Can you work these out from the model? Positions are in its coordinate system, mm. A direction names the side the tool comes from. Give positions to 0.01 mm unless a question says otherwise; leave off trailing zeros. Order: outer loops, then holes, each group sorted by start corner. A loop starts at its lowest first (then second) coordinate and runs counter-clockwise, first axis right, second up. Notation, with made-up numbers: (44.25, -19) -> (96.25, -19) arc R28 cw to (96.25, 8) -> close; hole circle Ø6 at (-40, 35.25). An arc over 180 degrees is marked (long way). Answer as a JSON object with one key per item and string values.
Autodesk Inventor part; units mm, degrees
ref_plane "YZ Plane" through (0, 0, 0) normal (1, 0, 0) x (0, 1, 0)
ref_plane "XZ Plane" through (0, 0, 0) normal (0, 1, 0) x (-1, 0, 0)
ref_plane "XY Plane" through (0, 0, 0) normal (0, 0, 1) x (1, 0, 0)
sketch "스케치1" plane through (0, 0, 0) normal (1, 0, 0) x (0, 1, 0)
  circle A0 centre (0, 0) radius 37
  circle A1 centre (0, 0) radius 4
  dimension "d0" = 74
  dimension "d1" = 8
extrude "돌출1" add sketch "스케치1" along normal blind 24
sketch "스케치2" plane through (24, 0, 0) normal (1, 0, 0) x (0, 0, -1)
  circle A0 centre (0, 0) radius 16
  dimension "d4" = 32
extrude "돌출2" cut sketch "스케치2" against normal blind 19
sketch "스케치4" plane through (5, 0, 0) normal (1, 0, 0) x (0, 0, -1)
  circle A0 centre (0, 10) radius 1.75
  circle A1 centre (10, 0) radius 1.75
  circle A2 centre (0, -10) radius 1.75
  circle A3 centre (-10, 0) radius 1.75
  point P0 (0, 0)
  dimension "d8" = 3.5
  dimension "d9" = 3.5
  dimension "d10" = 3.5
  dimension "d11" = 3.5
extrude "돌출3" cut sketch "스케치4" against normal blind 19
sketch "스케치5" plane through (24, 0, 0) normal (1, 0, 0) x (0, 0, -1)
  circle A0 centre (0, 0) radius 19
  circle A1 centre (0, 0) radius 32
  line L0 (-19.4142, 16.5858) -> (-14.7746, 11.9462)
  line L1 (-23.9974, 21.169) -> (-19.4142, 16.5858)
  line L2 (-16.5858, 19.4142) -> (-11.9462, 14.7746)
  line L3 (-16.5858, 19.4142) -> (-21.169, 23.9974)
  line L4 (16.5858, 19.4142) -> (11.9462, 14.7746)
  line L5 (16.5858, 19.4142) -> (21.169, 23.9974)
  line L6 (19.4142, 16.5858) -> (23.9974, 21.169)
  line L7 (19.4142, 16.5858) -> (14.7746, 11.9462)
  line L8 (16.5858, -19.4142) -> (11.9462, -14.7746)
  line L9 (16.5858, -19.4142) -> (21.169, -23.9974)
  line L10 (19.4142, -16.5858) -> (14.7746, -11.9462)
  line L11 (19.4142, -16.5858) -> (23.9974, -21.169)
  line L12 (-19.4142, -16.5858) -> (-14.7746, -11.9462)
  line L13 (-19.4142, -16.5858) -> (-23.9974, -21.169)
  line L14 (-16.5858, -19.4142) -> (-11.9462, -14.7746)
  line L15 (-16.5858, -19.4142) -> (-21.169, -23.9974)
  line L16 (-14.7746, -11.9462) -> (-23.9974, -21.169)
  dimension "d18" = 4
extrude "돌출4" cut sketch "스케치5" against normal blind 19 contours A0 L7 L6 A1 L11 L10 | A0 L2 L3 A1 L5 L4 | L8 L9 A1 L15 L14 A0 | A0 L12 L13 A1 L1 L0
sketch "스케치6" plane through (24, 0, 0) normal (1, 0, 0) x (0, 0, -1)
  circle A0 centre (0, 0) radius 35
  circle A1 centre (0, 0) radius 37
  dimension "d22" = 70
extrude "돌출5" cut sketch "스케치6" against normal blind 22
properties part number "바퀴8PI" material "아세탈 수지, 검은색"
1. Will these pins go through, and if not, where does the flat tip stop? pin 1 Ø4 at (x, z) = (4.5, 0.5) entering from -Y; pin 2 Ø3 at (x, y) = (10, -14) entering from +Z; pin 3 Ø6 at (x, z) = (16.5, 5.5) entering from -Y.
Worked answers:
{"pin 1": "y = -35", "pin 2": "z = 32.69", "pin 3": "y = -34.91"}
2. If we mould it in two halves opening along Z, with no side actions, what happens to faces 1 (the face through (14.63, -19.45, -16.62)), 2 (the face through (24, 5, -15.4))? For each: +Z half, -Z half, draft (parallel to the pull), parting line (faces both ways), or undercut.
Worked answers:
{"face 1": "undercut", "face 2": "draft"}
3. For faces 3 (the face through (2.535, 11.735, 0.228)), 4 (the face through (5, 24, 0)), which set-ups out of +Z, -Z, +X, -X, +Y, -Y let a thin tool reach every point of the face, with its end or its side?
Worked answers:
{"face 3": "+X, -X", "face 4": "+X"}
4. If we section it at C-C on x = 12.5: Please give me the cut outline in (y, z).
Worked answers:
{"outline": "circle Ø70 at (0, 0); hole (-24, -21.17) -> (-14.77, -11.95) arc R19 cw to (-14.77, 11.95) -> (-24, 21.17) arc R32 ccw to start; hole (-21.17, -24) arc R32 ccw to (21.17, -24) -> (11.95, -14.77) arc R19 cw to (-11.95, -14.77) -> close; hole (-21.17, 24) -> (-11.95, 14.77) arc R19 cw to (11.95, 14.77) -> (21.17, 24) arc R32 ccw to start; hole circle Ø32 at (0, 0); hole (14.77, -11.95) -> (24, -21.17) arc R32 ccw to (24, 21.17) -> (14.77, 11.95) arc R19 cw to start"}
5. Please list where these lines run through material, in increasing order: L1, parallel to Y at x = 1.9, z = 0; L2, parallel to Y at x = 2.6, z = 0; L3, parallel to Z at x = 5.25, y = 3.5.
Worked answers:
{"L1": "-37 to -11.75, -8.25 to -4, 4 to 8.25, 11.75 to 37", "L2": "-35 to -11.75, -8.25 to -4, 4 to 8.25, 11.75 to 35", "L3": "-34.82 to -31.81, -18.67 to -15.61, 15.61 to 18.67, 31.81 to 34.82"}
6. If we section it at D-D on z = 10: Please give me the cut outline in (x, y), then the cut area to 3 significant figures.
Worked answers:
{"outline": "(0, -35.62) -> (2, -35.62) -> (2, -33.54) -> (24, -33.54) -> (24, -30.4) -> (5, -30.4) -> (5, -16.16) -> (24, -16.16) -> (24, -12.49) -> (5, -12.49) -> (5, -1.75) -> (0, -1.75) -> close; (0, 1.75) -> (5, 1.75) -> (5, 12.49) -> (24, 12.49) -> (24, 16.16) -> (5, 16.16) -> (5, 30.4) -> (24, 30.4) -> (24, 33.54) -> (2, 33.54) -> (2, 35.62) -> (0, 35.62) -> close", "area": "585 mm²"}
7. If we section it at A-A on y = 0: Count the separate pieces of the cut face and the enclosed holes in it, then the cut area to 3 significant figures.
Worked answers:
{"separate pieces": "4", "enclosed holes": "0", "area": "511 mm²"}
